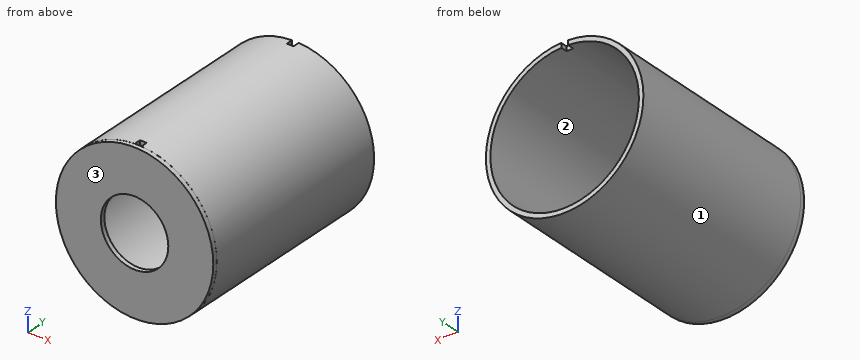
```python
from build123d import *

# Parameters (mm, degrees)
SKETCH1_R           = 88.9
SKETCH1_R_2         = 38.1
BOSS_EXTRUDE1_DEPTH = 5.08
SKETCH2_R           = 88.969872842
SKETCH2_R_2         = 83.889872842
BOSS_EXTRUDE2_DEPTH = 228.6
SKETCH3_W           = 7.62
SKETCH3_H           = 7.62
CUT_EXTRUDE1_DEPTH  = 89.969872842


with BuildPart() as part:
    # Sketch1 → Boss-Extrude1 (new body)
    with BuildSketch(Plane(origin=(0, 0, 0), x_dir=(1, 0, 0), z_dir=(0, 1, 0))):
        Circle(SKETCH1_R)
        Circle(SKETCH1_R_2, mode=Mode.SUBTRACT)
    extrude(amount=BOSS_EXTRUDE1_DEPTH)

    # Sketch2 → Boss-Extrude2 (add)
    with BuildSketch(Plane(origin=(0, 5.08, 0), x_dir=(1, 0, 0), z_dir=(0, 1, 0))):
        Circle(SKETCH2_R)
        Circle(SKETCH2_R_2, mode=Mode.SUBTRACT)
    extrude(amount=BOSS_EXTRUDE2_DEPTH)

    # Sketch3 → Cut-Extrude1 (cut, through all)
    with BuildSketch(Plane.XY):
        with Locations((0, 229.87)):
            Rectangle(SKETCH3_W, SKETCH3_H)
        with Locations((0, 8.89)):
            Rectangle(SKETCH3_W, SKETCH3_H)
    extrude(amount=CUT_EXTRUDE1_DEPTH, mode=Mode.SUBTRACT)


solid = part.part
```
Check sheet for the modelled part. Datum: model origin and axes. Units: mm. Face numbers are marked on the shaded views. Coordinates: 2 decimals unless noted, no trailing zeros. Write each loop counter-clockwise with the first axis right and the second up, starting at its lowest first coordinate (ties: lowest second). Pieces come first, ordered by that corner, then holes. Notation, with made-up numbers: (28, -21) - (80, -21) arc R16 ccw to (80, -17) - close; hole circle Ø4 at (-35.75, 35). An arc over 180 degrees is marked (long way). One line per question, with ' | ' between items.
Item 1: Sectioned sample at C-C on x = 21. Record the boundary of the cut face in (y, z).
Determined:
outline: (0, -86.38) - (5.08, -86.38) - (5.08, -86.46) - (233.68, -86.46) - (233.68, -81.22) - (5.08, -81.22) - (5.08, -31.79) - (0, -31.79) - close; (0, 31.79) - (5.08, 31.79) - (5.08, 81.22) - (233.68, 81.22) - (233.68, 86.46) - (5.08, 86.46) - (5.08, 86.38) - (0, 86.38) - close
Item 2: Sectioned sample at B-B on x = 0. Record the boundary of the cut face in (y, z), plus the area to 3 significant figures.
Determined:
outline: (0, -88.9) - (5.08, -88.9) - (5.08, -88.97) - (233.68, -88.97) - (233.68, -83.89) - (5.08, -83.89) - (5.08, -38.1) - (0, -38.1) - close; (0, 38.1) - (5.08, 38.1) - (5.08, 88.9) - (0, 88.9) - close; (12.7, 83.89) - (226.06, 83.89) - (226.06, 88.97) - (12.7, 88.97) - close | area: 2,760 mm2
Item 3: Thickness scan on line 1 (X direction, y = 3.1, z = 0); line 2 (Y direction, x = -21.5, z = -74). Record the ranges inside material, lowest first. Write a range as [from, to].
Determined:
line 1: x = [-88.9, -38.1], [38.1, 88.9] | line 2: y = [0, 5.08]
Item 4: Sectioned sample at D-D on y = 186.5. Record the boundary of the cut face in (x, z), plus the area to 3 significant figures.
Determined:
outline: circle Ø177.94 at (0, 0); hole circle Ø167.78 at (0, 0) | area: 2,760 mm2
Item 5: Gauge pin test, flat ends, axial feed: P1, Ø8, axis at x = 37, z = -62, coming from the +Y side; P2, Ø10, axis at y = 28.5, z = 8.5, coming from the +X side; P3, Ø2, axis at y = 88.5, z = -52.5, coming from the -X side. Record the tip position at first contact, or that the pin passes through.
Determined:
P1: stops at y = 5.08 | P2: stops at x = 88.9 | P3: stops at x = -72.55
Item 6: Sectioned sample at A-A on z = 0. Record the boundary of the cut face in (x, y).
Determined:
outline: (-88.97, 5.08) - (-88.9, 5.08) - (-88.9, 0) - (-38.1, 0) - (-38.1, 5.08) - (-83.89, 5.08) - (-83.89, 233.68) - (-88.97, 233.68) - close; (38.1, 0) - (88.9, 0) - (88.9, 5.08) - (88.97, 5.08) - (88.97, 233.68) - (83.89, 233.68) - (83.89, 5.08) - (38.1, 5.08) - close
Item 7: Mould release check, pull along Z, two halves, no side actions. Record for the marked faces 1, 2 and 3: pulls with the +Z half, pulls with the -Z half, needs draft (parallel to the pull), parting line crosses it, or undercut.
Determined:
face 1: parting line crosses it | face 2: undercut | face 3: needs draft
